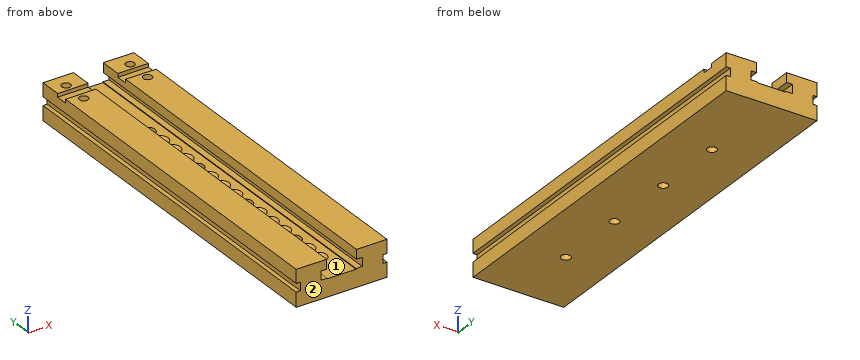
from build123d import *

# Parameters (mm, degrees)
BOSS_EXTRUDE1_DEPTH                      = 520
CUT_EXTRUDE1_REACH                       = 528.124
SKETCH4_W                                = 40
SKETCH4_H                                = 1
CBORE_FOR_M12_HEX_HEAD_BOLT1_D           = 13
CBORE_FOR_M12_HEX_HEAD_BOLT1_CBORE_D     = 19
CBORE_FOR_M12_HEX_HEAD_BOLT1_CBORE_DEPTH = 12
LPATTERN1_COUNT                          = 4
LPATTERN1_PITCH                          = 100
LPATTERN2_COUNT                          = 14
LPATTERN2_PITCH                          = 25
SKETCH7_W                                = 5
SKETCH7_H                                = 16
CUT_EXTRUDE2_DEPTH                       = 538.145231758
LPATTERN3_COUNT                          = 2
LPATTERN3_PITCH                          = 88
LPATTERN3_COUNT_DIR2                     = 2
LPATTERN3_PITCH_DIR2                     = 36


with BuildPart() as part:
    # Sketch1 → Boss-Extrude1 (new body)
    with BuildSketch(Plane(origin=(0, 0, 0), x_dir=(1, 0, 0), z_dir=(0, 1, 0))):
        Polygon((62.5, 0), (-62.5, 0), (-62.5, -20), (-56.7, -20), (-56.7, -31.5), (-62.5, -31.5), (-62.5, -50), (-20.5, -50), (-20.5, -37), (-28.5, -37), (-28.5, -25), (28.5, -25), (28.5, -37), (20.5, -37), (20.5, -50), (62.5, -50), (62.5, -31.5), (56.7, -31.5), (56.7, -20), (62.5, -20), align=None)
    extrude(amount=-BOSS_EXTRUDE1_DEPTH)

    # Sketch4 → Cut-Extrude1 (cut, up to next)
    with BuildSketch(Plane(origin=(0, 0, 0), x_dir=(1, 0, 0), z_dir=(0, 1, 0)), mode=Mode.PRIVATE) as cut_extrude1_sk1:
        with Locations((0, -24.5)):
            Rectangle(SKETCH4_W, SKETCH4_H)
    cut_extrude1_tool1 = extrude(cut_extrude1_sk1.sketch, amount=-CUT_EXTRUDE1_REACH, mode=Mode.PRIVATE) & part.part
    add(cut_extrude1_tool1.solids().sort_by_distance((0, 0, 24.5))[0], mode=Mode.SUBTRACT)

    # CBORE for M12 Hex Head Bolt1 (through all)
    with Locations(Plane.XY.offset(25)):
        with Locations((0, -122.5)):
            cbore_for_m12_hex_head_bolt1 = CounterBoreHole(CBORE_FOR_M12_HEX_HEAD_BOLT1_D / 2, CBORE_FOR_M12_HEX_HEAD_BOLT1_CBORE_D / 2, CBORE_FOR_M12_HEX_HEAD_BOLT1_CBORE_DEPTH)

    # LPattern1: CBORE for M12 Hex Head Bolt1 ×4
    with Locations(*[(0, -i * LPATTERN1_PITCH, 0) for i in range(1, LPATTERN1_COUNT)]):
        add(cbore_for_m12_hex_head_bolt1, mode=Mode.SUBTRACT)

    # Sketch6 → CSK for M10 Countersunk Flat Head Screw1 (revolve, cut)
    with BuildSketch(Plane(origin=(0, -147.5, 24), x_dir=(0, -1, 0), z_dir=(1, 0, 0))):
        Polygon((0, 0), (0, 14.304733405), (5.5, 11), (5.5, 5.5), (11, 0), align=None)
    csk_for_m10_countersunk_flat_head_screw1 = revolve(axis=Axis((0, -147.5, 30.35), (0, 0, -1)), mode=Mode.SUBTRACT)

    # LPattern2: CSK for M10 Countersunk Flat Head Screw1 ×14, 3 skipped
    with Locations(*[(0, -i * LPATTERN2_PITCH, 0) for i in range(1, LPATTERN2_COUNT) if i not in (3, 7, 11)]):
        add(csk_for_m10_countersunk_flat_head_screw1, mode=Mode.SUBTRACT)

    # Sketch7 → Cut-Extrude2 (cut, through all)
    with BuildSketch(Plane(origin=(62.5, 0, 0), x_dir=(0, 0, -1), z_dir=(1, 0, 0))):
        with Locations((-47.5, -38)):
            Rectangle(SKETCH7_W, SKETCH7_H)
    extrude(amount=-CUT_EXTRUDE2_DEPTH, mode=Mode.SUBTRACT)

    # Sketch9 → M14 Tapped Hole1 (revolve, cut)
    with BuildSketch(Plane(origin=(44, -20, 50), x_dir=(0, -1, 0), z_dir=(1, 0, 0))):
        Polygon((0, 0), (0, 39.605163714), (6, 36), (6, 0), align=None)
    m14_tapped_hole1 = revolve(axis=Axis((44, -20, 56.35), (0, 0, -1)), mode=Mode.SUBTRACT)

    # LPattern3: M14 Tapped Hole1 2 × 2
    with Locations(*[(-i * LPATTERN3_PITCH, -j * LPATTERN3_PITCH_DIR2, 0) for i in range(LPATTERN3_COUNT) for j in range(LPATTERN3_COUNT_DIR2) if (i, j) != (0, 0)]):
        add(m14_tapped_hole1, mode=Mode.SUBTRACT)


solid = part.part
The model under review builds one solid part; all positions refer to its coordinate system, in mm. Face numbers are marked on the shaded views. Give positions to 0.01 mm unless a question says otherwise; leave off trailing zeros. Write each loop counter-clockwise with the first axis right and the second up, starting at its lowest first coordinate (ties: lowest second). Pieces come first, ordered by that corner, then holes.
1. Add section B-B, the plane y = -92. Write out the cut boundary in (x, z), plus the area to 3 significant figures.
2. For P1, Ø2, axis at x = -6, y = -179.5, coming from the +Z side; P2, Ø9, axis at x = 0, y = -197.5, coming from the +Z side; P3, Ø17, axis at x = 0, y = -322.5, coming from the +Z side, all flat-tipped, find the tip position at first contact; note any pin that passes through.
3. Draft analysis for pull direction X (two halves, no side actions). For the marked faces 1 and 2, state which applies: +X half, -X half, draft (parallel to the pull), parting line (faces both ways), or undercut.
4. Wall thickness on L1, parallel to Y at x = 44, z = 27.5; L2, parallel to Z at x = 26, y = -275.5; L3, parallel to Y at x = 49, z = 35: over which ranges is each line inside the solid? List them lowest first.
Worked answers:
1. outline: (-62.5, 0) - (62.5, 0) - (62.5, 20) - (56.7, 20) - (56.7, 31.5) - (62.5, 31.5) - (62.5, 50) - (20.5, 50) - (20.5, 37) - (28.5, 37) - (28.5, 25) - (20, 25) - (20, 24) - (-20, 24) - (-20, 25) - (-28.5, 25) - (-28.5, 37) - (-20.5, 37) - (-20.5, 50) - (-62.5, 50) - (-62.5, 31.5) - (-56.7, 31.5) - (-56.7, 20) - (-62.5, 20) - close
1. area: 4,860 mm2
2. P1: stops at z = 23.22
2. P2: stops at z = 12.4
2. P3: stops at z = 13
3. face 1: undercut
3. face 2: draft
4. L1: y = -520 to -62, -50 to -26, -14 to 0
4. L2: z = 0 to 25, 37 to 50
4. L3: y = -520 to -59.32, -52.68 to -23.32, -16.68 to 0
